Check sheet for the drawn part. Datum: minimum x, y, z corner. Units: mm. A direction names the side the tool comes from. Coordinates: 2 decimals unless noted, no trailing zeros. Write each loop counter-clockwise with the first axis right and the second up, starting at its lowest first coordinate (ties: lowest second). Pieces come first, ordered by that corner, then holes. Notation, with made-up numbers: (-31, 39) -> (-5, 39) arc R11 cw to (-5, 49) -> close; hole circle Ø6 at (-33, 89). An arc over 180 degrees is marked (long way). Answer in a Markdown table with one row per item. Add a question column.
Q1. Section check D-D, the plane y = 0.75. Record the boundary of the cut face in (x, z) (1 decimal).
Q2. Section check B-B, the plane y = 4.2. Record the boundary of the cut face in (x, z) (1 decimal).
Q3. Section check A-A, the plane x = 3. Record the boundary of the cut face in (y, z).
Q4. Tool access check on the marked faces 4, 5 and 6. Record the directions out of +Z, -Z, +X, -X, +Y, -Y that give a thin tool (end or side, any length) a straight path to the whole face; none if there is none.
Q5. Thickness scan on line 1 (Z direction, x = 3, y = 2.45); line 2 (Y direction, x = 4.2, z = 1.75). Record the ranges inside material, lowest first.
Q6. Release check for a two-part mould opening along X. For the marked faces 1, 2 and 3 record: pulls with the +X half, pulls with the -X half, needs draft (parallel to the pull), parting line crosses it, or undercut.
Q7. Gauge pin test, flat ends, axial feed: P1, Ø1, axis at x = 5, y = 3, coming from the -Z side; P2, Ø2, axis at x = 2, z = 2.5, coming from the -Y side; P3, Ø1, axis at y = 2.5, z = 3, coming from the -X side; P4, Ø1.1, axis at x = 2.5, y = 4.5, coming from the -Z side. Record the tip position at first contact, or that the pin passes through.
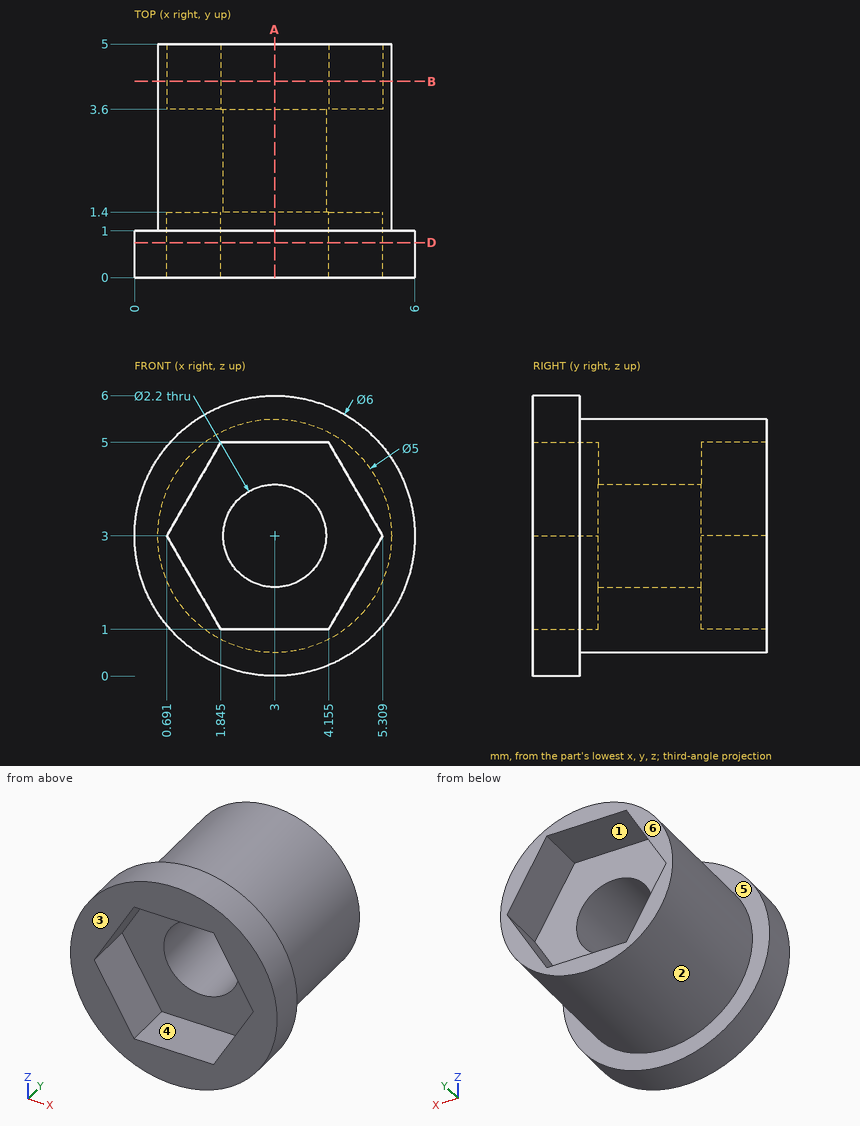
Calculated:
| question | item | result |
|---|---|---|
| 1 | outline | circle Ø6 at (3, 3); hole (0.7, 3) -> (1.8, 1) -> (4.2, 1) -> (5.3, 3) -> (4.2, 5) -> (1.8, 5) -> close |
| 2 | outline | circle Ø5 at (3, 3); hole (0.7, 3) -> (1.8, 1) -> (4.2, 1) -> (5.3, 3) -> (4.2, 5) -> (1.8, 5) -> close |
| 3 | outline | (0, 0) -> (1, 0) -> (1, 0.5) -> (5, 0.5) -> (5, 1) -> (3.6, 1) -> (3.6, 1.9) -> (1.4, 1.9) -> (1.4, 1) -> (0, 1) -> close; (0, 5) -> (1.4, 5) -> (1.4, 4.1) -> (3.6, 4.1) -> (3.6, 5) -> (5, 5) -> (5, 5.5) -> (1, 5.5) -> (1, 6) -> (0, 6) -> close |
| 4 | face 4 | -Y |
| 4 | face 5 | +Y |
| 4 | face 6 | +Z, -Z, +X, -X, +Y |
| 5 | line 1 | z = 0.5 to 1.9, 4.1 to 5.5 |
| 5 | line 2 | y = 1.4 to 3.6 |
| 6 | face 1 | undercut |
| 6 | face 2 | parting line crosses it |
| 6 | face 3 | needs draft |
| 7 | P1 | stops at z = 1 |
| 7 | P2 | stops at y = 0 |
| 7 | P3 | stops at x = 0.5 |
| 7 | P4 | stops at z = 0.5 |
